Here's how the part is built. I have some questions about the finished solid (model axes, mm). A direction names the side the tool comes from. Round coordinates to 2 decimals unless told otherwise and drop trailing zeros. Loops run counter-clockwise (first coordinate to the right, second up) from the corner with the lowest first, then second, coordinate; pieces in that order, holes last. Notation, with made-up numbers: (83, 79) - (100, 79) arc R23 cw to (100, 117) - close; hole circle Ø2 at (33, 86). An arc over 180 degrees is marked (long way). Answer as a JSON object with one key per item and string values. Group by question number.
1) I want a section at A-A, the plane x = 0. Please give me the cut outline in (y, z).
2) If we mould it in two halves opening along Z, with no side actions, what happens to faces 1 (the face through (0, -0.8, 1.6)), 2 (the face through (0, -1.55, 2)), 3 (the face through (0, -4.2, 7))? For each: pulls with the +Z half, pulls with the -Z half, needs draft (parallel to the pull), parting line crosses it, or undercut.
3) If I drill on line 1 along X through (y, z) = (-1.05, -2.5); line 2 along Z through (x, y) = (0, -2.15); line 3 along Z through (x, y) = (2, 2), over which ranges is the centre line in solid material (lowest first)? Write a range as [from, to].
4) Will these pins go through, and if not, where does the flat tip stop? P1, Ø4, axis at y = 3.5, z = -4, coming from the -X side; P2, Ø0.6, axis at x = 0, z = 5.5, coming from the -Y side; P3, Ø2, axis at x = -4, z = -2.5, coming from the -Y side; P4, Ø2, axis at x = 6.5, y = 2, coming from the +Z side (1 decimal).
5) I want a section at B-B, the plane y = -0.25. Please give me the cut outline in (x, z) (3 decimals).
6) Which directions (+Z, -Z, +X, -X, +Y, -Y) give clear straight access to the entire face, cutting with the end or side of a thin tool? Please do faces 4 (the face through (-0.369, -0.786, 8.892)), 5 (the face through (1.6, 0, -4)), 6 (the face through (4, -0.55, -2)), 7 (the face through (3, 0, 7)).
from build123d import *

# Parameters (mm, degrees)
CUT_EXTRUDE1_DEPTH      = 14.879571319
CUT_EXTRUDE1_DEPTH_BACK = 14.879571319
SKETCH3_R               = 1
CUT_EXTRUDE2_DEPTH      = 1


with BuildPart() as part:
    # Sketch1 → Revolve1 (revolve)
    with BuildSketch(Plane(origin=(0, 0, 0), x_dir=(0, 0, -1), z_dir=(1, 0, 0))):
        with BuildLine():
            Line((0, 0), (2.75, 0))
            Line((2.75, 0), (2.75, 4.3))
            Line((2.75, 4.3), (3.75, 4.3))
            Line((3.75, 4.3), (3.75, 3.5))
            ThreePointArc((3.75, 3.5), (4.775126266, 1.025126266), (7.25, 0))
            Line((7.25, 0), (8.9, 0))
            Line((8.9, 0), (8.9, -1.55))
            Line((8.9, -1.55), (7.45, -1.55))
            Line((7.45, -1.55), (7.45, -4.2))
            Line((7.45, -4.2), (6.65, -4.2))
            Line((6.65, -4.2), (6.65, -1.55))
            Line((6.65, -1.55), (0, -1.55))
            Line((0, -1.55), (0, 0))
        make_face()
    revolve(axis=Axis((0, -1.55, 0), (0, 1, 0)))

    # Sketch2 → Cut-Extrude1 (cut, two sides: drawn at the far end of the back side and taken through both)
    with BuildSketch(Plane.XZ.offset(1.55).offset(-CUT_EXTRUDE1_DEPTH_BACK)):
        with BuildLine():
            Line((1.6, 0), (1.6, -8.9))
            ThreePointArc((1.6, -8.9), (0, -10.5), (-1.6, -8.9))
            Line((-1.6, -8.9), (-1.6, 0))
            ThreePointArc((-1.6, 0), (0, 1.6), (1.6, 0))
        make_face()
    extrude(amount=CUT_EXTRUDE1_DEPTH + CUT_EXTRUDE1_DEPTH_BACK, mode=Mode.SUBTRACT)

    # Sketch3 → Cut-Extrude2 (cut)
    with BuildSketch(Plane.XZ.offset(1.55)):
        with Locations(Location((-4.330127019, -2.5, 0), (0, 0, 270))):
            Circle(SKETCH3_R)
        with Locations(Location((-4.330127019, 2.5, 0), (0, 0, 270))):
            Circle(SKETCH3_R)
        with Locations(Location((0, 5, 0), (0, 0, 270))):
            Circle(SKETCH3_R)
        with Locations(Location((4.330127019, 2.5, 0), (0, 0, 270))):
            Circle(SKETCH3_R)
        with Locations(Location((4.330127019, -2.5, 0), (0, 0, 270))):
            Circle(SKETCH3_R)
        with Locations((0, -5)):
            Circle(SKETCH3_R)
    extrude(amount=-CUT_EXTRUDE2_DEPTH, mode=Mode.SUBTRACT)


solid = part.part
Outcome:
{
 "1": {"outline": "(-4.2, 6.65) - (-1.55, 6.65) - (-1.55, 6) - (-0.55, 6) - (-0.55, 4) - (-1.55, 4) - (-1.55, 1.6) - (0, 1.6) - (0, 2.75) - (4.3, 2.75) - (4.3, 3.75) - (3.5, 3.75) arc R3.5 cw to (0, 7.25) - (0, 8.9) - (-1.55, 8.9) - (-1.55, 7.45) - (-4.2, 7.45) - close"},
 "2": {"face 1": "pulls with the -Z half", "face 2": "undercut", "face 3": "needs draft"},
 "3": {"line 1": "[-8.54, -5.33], [-3.33, -1.6], [1.6, 3.33], [5.33, 8.54]", "line 2": "[6.65, 7.45]", "line 3": "[-3.57, -1.89], [1.89, 3.57]"},
 "4": {"P1": "x = -3.17", "P2": "y = -0.55", "P3": "y = -1.55", "P4": "through"},
 "5": {"outline": "(-1.6, -8.755) - (-1.6, 0) arc R1.6 cw to (1.6, 0) - (1.6, -8.755) arc R8.9 ccw (long way) to start"},
 "6": {"face 4": "+Y, -Y", "face 5": "-Z, +Y, -Y", "face 6": "-Y", "face 7": "+Y"}
}
